```python
from build123d import *

# Parameters (mm, degrees)
SKETCH_1_W          = 74.5
SKETCH_1_H          = 166.2
EXTRUDE_1_DEPTH     = 4.9
SKETCH_3_W          = 74.5
SKETCH_3_H          = 5.95
EXTRUDE_2_DEPTH     = 8.3
SKETCH_4_W          = 25
SKETCH_4_H          = 0.2
EXTRUDE_4_DEPTH     = 10.5
SKETCH_6_W          = 25
SKETCH_6_H          = 0.2
EXTRUDE_5_DEPTH     = 7.9
SKETCH_7_W          = 25
SKETCH_7_H          = 0.2
EXTRUDE_6_DEPTH     = 7.9
SKETCH_8_W          = 4.335096154
SKETCH_8_H          = 0.488461538
CUT_EXTRUDE_1_DEPTH = 0.1


with BuildPart() as part:
    # 草图1 → 凸台-拉伸1 (new, symmetric)
    with BuildSketch(Plane.XY):
        Rectangle(SKETCH_1_W, SKETCH_1_H)
    extrude(amount=EXTRUDE_1_DEPTH, both=True)

    # 草图3 → 凸台-拉伸2 (add)
    with BuildSketch(Plane(origin=(0, 83.1, 0), x_dir=(1, 0, 0), z_dir=(0, 1, 0))):
        with Locations((0, 1.925)):
            Rectangle(SKETCH_3_W, SKETCH_3_H)
    extrude(amount=EXTRUDE_2_DEPTH)

    # 草图4 → 凸台-拉伸4 (add)
    with BuildSketch(Plane(origin=(0, 83.1, 0), x_dir=(1, 0, 0), z_dir=(0, 1, 0))):
        with Locations((-19, -1.85)):
            Rectangle(SKETCH_4_W, SKETCH_4_H)
        with Locations((19, -1.85)):
            Rectangle(SKETCH_4_W, SKETCH_4_H)
    extrude(amount=EXTRUDE_4_DEPTH)

    # 草图6 → 凸台-拉伸5 (add)
    with BuildSketch(Plane.XY.offset(1.95)):
        with Locations((-19, 93.5)):
            Rectangle(SKETCH_6_W, SKETCH_6_H)
    extrude(amount=EXTRUDE_5_DEPTH)

    # 草图7 → 凸台-拉伸6 (add)
    with BuildSketch(Plane(origin=(0, 0, 1.75), x_dir=(-1, 0, 0), z_dir=(0, 0, -1))):
        with Locations((-19, 93.5)):
            Rectangle(SKETCH_7_W, SKETCH_7_H)
    extrude(amount=EXTRUDE_6_DEPTH)

    # 草图8 → 切除-拉伸1 (cut)
    with BuildSketch(Plane(origin=(0, 0, -4.9), x_dir=(-1, 0, 0), z_dir=(0, 0, -1))):
        Polygon((-19.751628191, 76.72094721), (-19.751628191, 78.125274133), (-18.713647422, 78.125274133), (-18.713647422, 76.72094721), (-15.416532037, 76.72094721), (-15.416532037, 76.293543364), (-18.713647422, 76.293543364), (-18.713647422, 74.889216441), (-19.751628191, 74.889216441), (-19.751628191, 76.293543364), (-23.048743575, 76.293543364), (-23.048743575, 76.72094721), align=None)
        with Locations((14.959669886, 75.988254902)):
            Rectangle(SKETCH_8_W, SKETCH_8_H)
    cut_extrude_1 = extrude(amount=-CUT_EXTRUDE_1_DEPTH, mode=Mode.SUBTRACT)

    # 镜向1: 切除-拉伸1 across plane
    add(cut_extrude_1.mirror(Plane.XY), mode=Mode.SUBTRACT)


solid = part.part
```
Work out the finished part from the listing and answer in its coordinate system (mm). A direction names the side the tool comes from. Give positions to 0.01 mm unless a question says otherwise; leave off trailing zeros. Write each loop counter-clockwise with the first axis right and the second up, starting at its lowest first coordinate (ties: lowest second). Pieces come first, ordered by that corner, then holes.
(1) The part is cut by section B-B on z = 6.5. Write down the section's boundary in (x, y), plus the area to 3 significant figures.
Final values:
outline: (-31.5, 93.4) - (-6.5, 93.4) - (-6.5, 93.6) - (-31.5, 93.6) - close
area: 5.00 mm2
(2) The mould has two halves that part along Y. Classify faces 5 (the flat face through (19, 93.6, -2)), 6 (the flat face through (19, 93.4, -2)), 7 (the flat face through (-1, -83.1, 0)): pulls with the +Y half, pulls with the -Y half, needs draft (parallel to the pull), parting line crosses it, or undercut.
Final values:
face 5: pulls with the +Y half
face 6: undercut
face 7: pulls with the -Y half
(3) The part is cut by section D-D on x = 3.5. Write down the section's boundary in (y, z).
Final values:
outline: (-83.1, -4.9) - (91.4, -4.9) - (91.4, 1.05) - (83.1, 1.05) - (83.1, 4.9) - (-83.1, 4.9) - close
(4) The part is cut by section C-C on y = -57. Write down the section's boundary in (x, z), plus the area to 3 significant figures.
Final values:
outline: (-37.25, -4.9) - (37.25, -4.9) - (37.25, 4.9) - (-37.25, 4.9) - close
area: 730 mm2
(5) Straight lines are drawn through the part: line 1 (Y direction, x = 14, z = -2.5); line 2 (Z direction, x = 28, y = -20); line 3 (Y direction, x = -10, z = 8). For each, find the intervals that lie inside material, in ascending order.
Final values:
line 1: y = -83.1 to 91.4, 93.4 to 93.6
line 2: z = -4.9 to 4.9
line 3: y = 93.4 to 93.6
(6) Flat-ended cylindrical pins translate along their axes: pin 1 Ø4 at (x, y) = (2.5, 86) entering from +Z; pin 2 Ø3 at (y, z) = (38.5, 6) entering from +X; pin 3 Ø4 at (x, y) = (-2.5, -44.5) entering from -Z; pin 4 Ø12 at (x, y) = (-20, 16.5) entering from +Z. Find the tip coordinate at first contact, or state that the pin passes through.
Final values:
pin 1: stops at z = 1.05
pin 2: stops at x = 37.25
pin 3: stops at z = -4.9
pin 4: stops at z = 4.9
(7) The part is cut by section A-A on x = 26.5. Write down the section's boundary in (y, z).
Final values:
outline: (-83.1, -4.9) - (91.4, -4.9) - (91.4, 1.05) - (83.1, 1.05) - (83.1, 1.75) - (93.4, 1.75) - (93.4, -6.15) - (93.6, -6.15) - (93.6, 1.95) - (83.1, 1.95) - (83.1, 4.9) - (-83.1, 4.9) - close
(8) Which of the six approach directions +Z, -Z, +X, -X, +Y, -Y give full straight-line access (tool end or side, diameter ignored) to faces 1 (the flat face through (-1, 91.4, -2)), 2 (the flat face through (-1, 3, -4.9)), 3 (the flat face through (-1, 87, 1.05)), 4 (the flat face through (-19, 93.4, 6))?
Final values:
face 1: -Z, +X, -X
face 2: -Z, +X, -X, -Y
face 3: +X, -X
face 4: +Z, +X, -X
